Geometry: final body of the model. Coordinates: model frame, mm. Face numbers are marked on the shaded views. A direction names the side the tool comes from. Give positions to 0.01 mm unless a question says otherwise; leave off trailing zeros. Write each loop counter-clockwise with the first axis right and the second up, starting at its lowest first coordinate (ties: lowest second). Pieces come first, ordered by that corner, then holes. Notation, with made-up numbers: (-4, -12.5) - (28, -12.5) arc R17 ccw to (28, -6.5) - close; hole circle Ø11 at (74.5, 27.25). An arc over 180 degrees is marked (long way). Return JSON: item names as keys, results as strings.
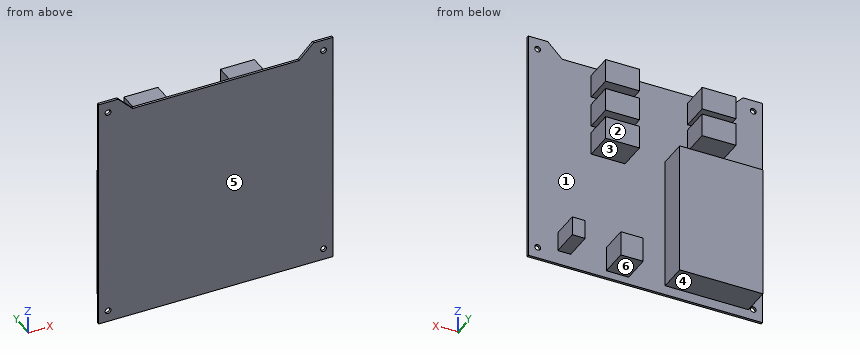
from build123d import *

# Parameters (mm, degrees)
SKETCH1_R           = 1.905
BOSS_EXTRUDE1_DEPTH = 1.5875
SKETCH2_W           = 22.225
SKETCH2_H           = 15.24
SKETCH2_W_2         = 14.620181031
SKETCH2_H_2         = 16.374602754
SKETCH2_W_3         = 54.61
SKETCH2_H_3         = 87.63
SKETCH2_W_4         = 8.479704998
SKETCH2_H_4         = 12.573355687
BOSS_EXTRUDE2_DEPTH = 18.542


with BuildPart() as part:
    # Sketch1 → Boss-Extrude1 (new body)
    with BuildSketch(Plane(origin=(0, 0, 0), x_dir=(1, 0, 0), z_dir=(0, 1, 0))):
        Polygon((-76.835, 77.47), (76.835, 77.47), (76.835, -77.47), (64.135, -77.47), (54.61, -67.945), (-54.61, -67.945), (-64.135, -77.47), (-76.835, -77.47), align=None)
        with Locations(Location((-70.739, 70.0405, 0), (0, 0, 270))):
            Circle(SKETCH1_R, mode=Mode.SUBTRACT)
        with Locations(Location((-70.739, -70.0405, 0), (0, 0, 270))):
            Circle(SKETCH1_R, mode=Mode.SUBTRACT)
        with Locations(Location((70.739, -70.0405, 0), (0, 0, 270))):
            Circle(SKETCH1_R, mode=Mode.SUBTRACT)
        with Locations(Location((70.739, 70.0405, 0), (0, 0, 270))):
            Circle(SKETCH1_R, mode=Mode.SUBTRACT)
    extrude(amount=BOSS_EXTRUDE1_DEPTH)

    # Sketch2 → Boss-Extrude2 (add)
    with BuildSketch(Plane(origin=(0, 1.5875, 0), x_dir=(1, 0, 0), z_dir=(0, 1, 0))):
        with Locations((-38.837784726, -54.764880682)):
            Rectangle(SKETCH2_W, SKETCH2_H)
        with Locations((-38.837784726, -35.904847152)):
            Rectangle(SKETCH2_W, SKETCH2_H)
        with Locations((24.469923971, -54.764880682)):
            Rectangle(SKETCH2_W, SKETCH2_H)
        with Locations((24.469923971, -34.296627238)):
            Rectangle(SKETCH2_W, SKETCH2_H)
        with Locations((24.469923971, -14.413181036)):
            Rectangle(SKETCH2_W, SKETCH2_H)
        with Locations((18.328285521, 64.38959472)):
            Rectangle(SKETCH2_W_2, SKETCH2_H_2)
        with Locations((-40.291302772, 27.368792631)):
            Rectangle(SKETCH2_W_3, SKETCH2_H_3)
        with Locations((53.270518185, 61.904163944)):
            Rectangle(SKETCH2_W_4, SKETCH2_H_4)
    extrude(amount=BOSS_EXTRUDE2_DEPTH)


solid = part.part
Q1. Set-up query: the marked faces 3, 4, 5 and 6. Return all of +Z, -Z, +X, -X, +Y, -Y with unobstructed straight access to the full face (end or side cutting, diameter ignored); none if empty.
Answer key:
{"face 3": "+X, +Y", "face 4": "-Z, -X, +Y", "face 5": "+Z, -Z, +X, -X, -Y", "face 6": "-Z, +X, -X, +Y"}
Q2. Pin query (flat end, axial travel): P1, Ø7, axis at x = 55, y = 14, coming from the -Z side; P2, Ø8, axis at y = 13.5, z = -62.5, coming from the -X side; P3, Ø7.5, axis at x = 17.5, y = 8, coming from the +Z side. Return the tip coordinate at first contact, or that it passes through.
Answer key:
{"P1": "stops at z = -68.19", "P2": "stops at x = -67.6", "P3": "stops at z = 62.38"}
Q3. Section query A-A, the plane y = 8.5. Count the separate pieces of the cut face and the enclosed holes in it, plus the area to 3 significant figures.
Answer key:
{"separate pieces": "8", "enclosed holes": "0", "area": "6,830 mm^2"}
Q4. Section query D-D, the plane x = -61. Return the cut outline in (y, z) (1 decimal), plus the area to 3 significant figures.
Answer key:
{"outline": "(0, -77.5) - (1.6, -77.5) - (1.6, -71.2) - (20.1, -71.2) - (20.1, 16.4) - (1.6, 16.4) - (1.6, 74.3) - (0, 74.3) - close", "area": "1,870 mm^2"}
Q5. Section query B-B, the plane z = -52. Return the cut outline in (x, y) (1 decimal), plus the area to 3 significant figures.
Answer key:
{"outline": "(-76.8, 0) - (76.8, 0) - (76.8, 1.6) - (-13, 1.6) - (-13, 20.1) - (-67.6, 20.1) - (-67.6, 1.6) - (-76.8, 1.6) - close", "area": "1,260 mm^2"}
Q6. Mould query, pull axis X, two halves, no side actions, for the marked faces 1 and 2. Classes: pulls with the +X half, pulls with the -X half, needs draft (parallel to the pull), parting line crosses it, or undercut.
Answer key:
{"face 1": "undercut", "face 2": "needs draft"}
Q7. Material intervals for probe 1 along X at (y, z) = (2.5, -57); probe 2 along Z at (x, y) = (32, 1.75); probe 3 along Z at (x, y) = (-28.5, 8.5), sorted ascending. Write a range as [from, to].
Answer key:
{"probe 1": "x = [-67.6, -12.99], [11.02, 25.64], [49.03, 57.51]", "probe 2": "z = [6.79, 22.03], [26.68, 41.92], [47.14, 62.38]", "probe 3": "z = [-71.18, 16.45], [28.28, 43.52], [47.14, 62.38]"}
Q8. Section query C-C, the plane x = -29.5. Return the cut outline in (y, z) (1 decimal).
Answer key:
{"outline": "(0, -77.5) - (1.6, -77.5) - (1.6, -71.2) - (20.1, -71.2) - (20.1, 16.4) - (1.6, 16.4) - (1.6, 28.3) - (20.1, 28.3) - (20.1, 43.5) - (1.6, 43.5) - (1.6, 47.1) - (20.1, 47.1) - (20.1, 62.4) - (1.6, 62.4) - (1.6, 67.9) - (0, 67.9) - close"}
